```python
from build123d import *

# Parameters (mm, degrees)
SKETCH1_W           = 25
SKETCH1_H           = 20
BOSS_EXTRUDE1_DEPTH = 22
FILLET1_RADIUS      = 10
FILLET1_LENGTH      = 22
SKETCH2_R           = 5
BOSS_EXTRUDE2_DEPTH = 30
SKETCH3_R           = 3
CUT_EXTRUDE1_DEPTH  = 30
SKETCH4_W           = 5
SKETCH4_H           = 34
CUT_EXTRUDE2_DEPTH  = 31


with BuildPart() as part:
    # Sketch1 → Boss-Extrude1 (new body)
    with BuildSketch(Plane(origin=(0, 0, 0), x_dir=(0, 0, -1), z_dir=(1, 0, 0))):
        with Locations((12.5, 10)):
            Rectangle(SKETCH1_W, SKETCH1_H)
    extrude(amount=BOSS_EXTRUDE1_DEPTH)

    # Fillet1: full round fillet: the end face becomes a half cylinder, R = half its width
    fillet1_face = Plane((11, 10, 0), x_dir=(-1, 0, 0), z_dir=(0, 0, 1))  # on the end face: x along it, z out of the body
    fillet1_slab = fillet1_face.offset(-FILLET1_RADIUS / 2) * Box(FILLET1_LENGTH, 2 * FILLET1_RADIUS, FILLET1_RADIUS, mode=Mode.PRIVATE)  # the body's end, R deep
    fillet1_round = Plane((11, 10, -10), x_dir=(0, 0, 1), z_dir=(-1, 0, 0)) * Cylinder(FILLET1_RADIUS, FILLET1_LENGTH, mode=Mode.PRIVATE)  # its axis R under the face
    add(fillet1_slab - fillet1_round, mode=Mode.SUBTRACT)

    # Sketch2 → Boss-Extrude2 (add)
    with BuildSketch(Plane(origin=(0, 0, -25), x_dir=(-1, 0, 0), z_dir=(0, 0, -1))):
        with Locations(Location((-11, 10, 0), (0, 0, 180))):
            Circle(SKETCH2_R)
    extrude(amount=BOSS_EXTRUDE2_DEPTH)

    # Sketch3 → Cut-Extrude1 (cut)
    with BuildSketch(Plane(origin=(22, 0, 0), x_dir=(0, 0, -1), z_dir=(1, 0, 0))):
        with Locations((10, 10)):
            Circle(SKETCH3_R)
    extrude(amount=-CUT_EXTRUDE1_DEPTH, mode=Mode.SUBTRACT)

    # Sketch4 → Cut-Extrude2 (cut)
    with BuildSketch(Plane(origin=(0, 20, 0), x_dir=(1, 0, 0), z_dir=(0, 1, 0))):
        with Locations((11, 0)):
            Rectangle(SKETCH4_W, SKETCH4_H)
    extrude(amount=-CUT_EXTRUDE2_DEPTH, mode=Mode.SUBTRACT)


solid = part.part
```
Geometry: final body of the model. Coordinates: model frame, mm. A direction names the side the tool comes from. Coordinates: 2 decimals unless noted, no trailing zeros. Order: outer loops, then holes, each group sorted by start corner. A loop starts at its lowest first (then second) coordinate and runs counter-clockwise, first axis right, second up. Notation, with made-up numbers: (43, 40.5) - (62, 40.5) arc R20 cw to (62, 76.5) - close; hole circle Ø11 at (44.25, 84). An arc over 180 degrees is marked (long way). Return JSON: item names as keys, results as strings. Group by question number.
1. Cut plane C-C (x = 11). Output: boundary loops of the cut face in (y, z), plus the area to 3 significant figures.
2. Material intervals for line 1 along Y through (x, z) = (3.5, -10); line 2 along X through (y, z) = (17, -8); line 3 along Z through (x, y) = (13, 13.75), sorted ascending. Write a range as [from, to].
3. Set-up query: faces 1 (the face through (22, 10, -15)), 2 (the face through (11, 10, -17)), 3 (the face through (8, 5, -25)). Return all of +Z, -Z, +X, -X, +Y, -Y with unobstructed straight access to the full face (end or side cutting, diameter ignored); none if empty.
4. Cut plane D-D (x = 17.75). Output: boundary loops of the cut face in (y, z), plus the area to 3 significant figures.
5. Pin query (flat end, axial travel): pin 1 (12 mm diameter, centred on x = 8.5, z = -47.5, fed in from +Y); pin 2 (1.5 mm diameter, centred on y = 15, z = -45.5, fed in from +X); pin 3 (4 mm diameter, centred on x = 10, y = 5.5, fed in from +Z); pin 4 (4 mm diameter, centred on x = 2.5, z = -40.5, fed in from +Y). Return the tip coordinate at first contact, or that it passes through.
6. Cut plane B-B (z = -14). Output: boundary loops of the cut face in (x, y), plus the area to 3 significant figures.
7. Pull-direction query (X, two-part tool) for faces 4 (the face through (13.5, 10, -6)), 5 (the face through (8.5, 10, -6)), 6 (the face through (15.77, 8.5, -39.79)), 7 (the face through (4, 10, 0)); classes: pulls with the +X half, pulls with the -X half, needs draft (parallel to the pull), parting line crosses it, or undercut.
8. Cut plane A-A (y = 10). Output: boundary loops of the cut face in (x, z).
Resolved:
{
 "1": {"outline": "(0, -25) - (5, -25) - (5, -55) - (15, -55) - (15, -25) - (20, -25) - (20, -17) - (0, -17) - close", "area": "460 mm²"},
 "2": {"line 1": "y = [0, 7], [13, 20]", "line 2": "x = [0, 8.5], [13.5, 22]", "line 3": "z = [-55, -17]"},
 "3": {"face 1": "+Z, -Z, +X, +Y, -Y", "face 2": "+Z, +Y, -Y", "face 3": "-Z"},
 "4": {"outline": "(0, -25) - (20, -25) - (20, -10) arc R10 ccw to (0, -10) - close; hole circle Ø6 at (10, -10)", "area": "429 mm²"},
 "5": {"pin 1": "stops at y = 15", "pin 2": "stops at x = 13.63", "pin 3": "stops at z = -0.52", "pin 4": "passes through"},
 "6": {"outline": "(0, 0) - (8.5, 0) - (8.5, 20) - (0, 20) - close; (13.5, 0) - (22, 0) - (22, 20) - (13.5, 20) - close", "area": "340 mm²"},
 "7": {"face 4": "undercut", "face 5": "undercut", "face 6": "parting line crosses it", "face 7": "needs draft"},
 "8": {"outline": "(0, -25) - (6, -25) - (6, -55) - (16, -55) - (16, -25) - (22, -25) - (22, -13) - (13.5, -13) - (13.5, -17) - (8.5, -17) - (8.5, -13) - (0, -13) - close; (0, -7) - (8.5, -7) - (8.5, 0) - (0, 0) - close; (13.5, -7) - (22, -7) - (22, 0) - (13.5, 0) - close"}
}
